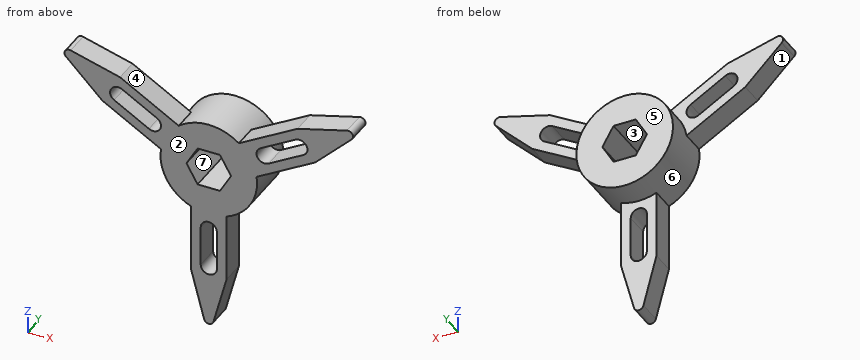
```python
from build123d import *

# Parameters (mm, degrees)
SKETCH1_R           = 30
BOSS_EXTRUDE1_DEPTH = 32
BOSS_EXTRUDE2_DEPTH = 15
CIRPATTERN2_COUNT   = 3


with BuildPart() as part:
    # Sketch1 → Boss-Extrude1 (new body)
    with BuildSketch(Plane(origin=(0, 0, 0), x_dir=(1, 0, 0), z_dir=(0, 1, 0))):
        with Locations(Location((0, 0, 0), (0, 0, 270))):
            Circle(SKETCH1_R)
        Polygon((6.92820323, -12), (13.856406461, 0), (6.92820323, 12), (-6.92820323, 12), (-13.856406461, 0), (-6.92820323, -12), align=None, mode=Mode.SUBTRACT)
    extrude(amount=BOSS_EXTRUDE1_DEPTH)

    # Sketch1<3> → Boss-Extrude2 (add)
    with BuildSketch(Plane(origin=(0, 0, 0), x_dir=(1, 0, 0), z_dir=(0, 1, 0))):
        with BuildLine():
            Line((11, 27.910571474), (11, 70))
            Line((11, 70), (2.901151097, 100.763755402))
            ThreePointArc((2.901151097, 100.763755402), (0, 103), (-2.901151097, 100.763755402))
            Line((-2.901151097, 100.763755402), (-11, 70))
            Line((-11, 70), (-11, 27.910571474))
            ThreePointArc((-11, 27.910571474), (0, 30), (11, 27.910571474))
        make_face()
        with BuildLine():
            ThreePointArc((5, 40), (0, 35), (-5, 40))
            Line((-5, 40), (-5, 65))
            ThreePointArc((-5, 65), (0, 70), (5, 65))
            Line((5, 65), (5, 40))
        make_face(mode=Mode.SUBTRACT)
    extrude(amount=BOSS_EXTRUDE2_DEPTH)


with BuildPart() as cirpattern2_1:
    # CirPattern2: pattern copy
    add(part.part.rotate(Axis((0, 0, 0), (0, 1, 0)), 1 * 360 / CIRPATTERN2_COUNT))


with BuildPart() as cirpattern2_2:
    # CirPattern2: pattern copy
    add(part.part.rotate(Axis((0, 0, 0), (0, 1, 0)), 2 * 360 / CIRPATTERN2_COUNT))

    # Combine2: read off the stored shape, not the designer's step
    # Combine2: union part, CirPattern2_1
    add(part.part)
    add(cirpattern2_1.part)


solid = cirpattern2_2.part
```
Input: part model. Units: mm. Frame: model coordinates. Face numbers are marked on the shaded views. A direction names the side the tool comes from. Round coordinates to 2 decimals unless told otherwise and drop trailing zeros. Loops run counter-clockwise (first coordinate to the right, second up) from the corner with the lowest first, then second, coordinate; pieces in that order, holes last. Notation, with made-up numbers: M 29.5,7 L 33.5,7 A26 ccw 33.5,46 Z; hole C 9.25,-2.75 d9. An arc over 180 degrees is marked long. Answer in a Markdown table with one row per item. Add a question column.
1. Section A-A (z = -54). Output: boundary loops of the cut face in (x, y).
2. Section D-D (y = 10.5). Give the number of separate pieces and of enclosed holes in the cut face, and give its area (3 significant figures).
3. Section C-C (z = 20). Output: boundary loops of the cut face in (x, y).
4. Set-up query: the marked faces 4, 5, 6 and 7. Return all of +Z, -Z, +X, -X, +Y, -Y with unobstructed straight access to the full face (end or side cutting, diameter ignored); none if empty.
5. Ray query, probe 1 along X at (y, z) = (10, -62); probe 2 along Z at (x, y) = (-44, 10); probe 3 along X at (y, z) = (9, 1.5). Return the intervals inside material, ascending.
6. Contact query for flat-ended pins moving along their axis: pin 1 (10 mm diameter, centred on y = 25.5, z = 26, fed in from +X); pin 2 (10 mm diameter, centred on y = 21, z = 5.5, fed in from -X); pin 3 (8 mm diameter, centred on y = 8.5, z = -14.5, fed in from +X). Output: stop coordinate, or through.
7. Mould query, pull axis Z, two halves, no side actions, for the marked faces 1, 2 and 3. Classes: released by +Z, released by -Z, zero draft, split by the parting line, or undercut.
8. Section B-B (x = 51). Output: boundary loops of the cut face in (y, z).
Values follow:
| question | item | result |
|---|---|---|
| 1 | outline | M -11,0 L -5,0 L -5,15 L -11,15 Z; M 5,0 L 11,0 L 11,15 L 5,15 Z |
| 2 | separate pieces | 1 |
| 2 | enclosed holes | 4 |
| 2 | area | 5,340 mm^2 |
| 3 | outline | M -56.64,0 L -44.64,0 L -44.64,15 L -56.64,15 Z; M -29.64,0 L 29.64,0 L 29.64,15 L 22.36,15 L 22.36,32 L -22.36,32 L -22.36,15 L -29.64,15 Z; M 44.64,0 L 56.64,0 L 56.64,15 L 44.64,15 Z |
| 4 | face 4 | +Z, +Y, -Y |
| 4 | face 5 | +Z, -Z, +X, -X, +Y |
| 4 | face 6 | +Y |
| 4 | face 7 | +Y, -Y |
| 5 | probe 1 | -11 to -5, 5 to 11 |
| 5 | probe 2 | 12.7 to 19.63, 31.18 to 38.11 |
| 5 | probe 3 | -29.96 to -12.99, 12.99 to 29.96 |
| 6 | pin 1 | x = 21.42 |
| 6 | pin 2 | x = -30 |
| 6 | pin 3 | x = 28.1 |
| 7 | face 1 | released by -Z |
| 7 | face 2 | zero draft |
| 7 | face 3 | undercut |
| 8 | outline | M 0,16.74 L 15,16.74 L 15,23.67 L 0,23.67 Z; M 0,35.22 L 15,35.22 L 15,42.15 L 0,42.15 Z |
